```python
from build123d import *

# Parameters (mm, degrees)
SKETCH1_R           = 3.9
BOSS_EXTRUDE1_DEPTH = 50
SKETCH1_3_R         = 9.9
SKETCH1_3_R_2       = 3.9
BOSS_EXTRUDE2_DEPTH = 3
FILLET1_R           = 1


with BuildPart() as part:
    # Sketch1 → Boss-Extrude1 (new body)
    with BuildSketch(Plane.XY):
        Circle(SKETCH1_R)
    extrude(amount=BOSS_EXTRUDE1_DEPTH)

    # Sketch1_3 → Boss-Extrude2 (add)
    with BuildSketch(Plane.XY):
        Circle(SKETCH1_3_R)
        Circle(SKETCH1_3_R_2, mode=Mode.SUBTRACT)
        Circle(SKETCH1_3_R_2)
    extrude(amount=-BOSS_EXTRUDE2_DEPTH)

    # Fillet1
    fillet1_edges = [part.edges().sort_by_distance(p)[0] for p in [
        (-3.9, 0, 0),
    ]]
    fillet(fillet1_edges, radius=FILLET1_R)


solid = part.part
```
Can you work these out from the model? Positions are in its coordinate system, mm. A direction names the side the tool comes from. Give positions to 0.01 mm unless a question says otherwise; leave off trailing zeros. Write each loop counter-clockwise with the first axis right and the second up, starting at its lowest first coordinate (ties: lowest second). Pieces come first, ordered by that corner, then holes. Notation, with made-up numbers: (32.5, -1.75) - (36.5, -1.75) arc R36 cw to (36.5, 36.25) - close; hole circle Ø8 at (33, 49). An arc over 180 degrees is marked (long way). Write item = value, one per line. Start each with the question number.
1. Imagine slicing it at D-D (y = -5.5). Please give me the cut outline in (x, z).
2. Imagine slicing it at A-A (y = 0). Please give me the cut outline in (x, z), and give its area (3 significant figures).
3. Imagine slicing it at C-C (z = 18). Please give me the cut outline in (x, y), and give its area (3 significant figures).
4. Please list where these lines run through material, in increasing order: line 1 (Z direction, x = -6.5, y = -6.5); line 2 (Y direction, x = 0, z = 38.5); line 3 (X direction, y = 0.25, z = 26).
5. On a 3-axis mill with a long thin cutter (end or side, diameter ignored), from which of +Z, -Z, +X, -X, +Y, -Y can I reach the whole of each face in a straight line? I mean faces 1 (the face through (-5, -2, 0)), 2 (the face through (9.443, 2.974, -1.479)). Say none if no direction works.
6. For pin 1 (2 mm diameter, centred on x = 3, z = 19, fed in from +Y); pin 2 (3 mm diameter, centred on x = -3, z = 39, fed in from +Y); pin 3 (6 mm diameter, centred on y = 6, z = 42, fed in from -X), each with a flat end and sliding along its axis, tell me the tip position at first contact or that it passes through.
Worked answers:
q1.outline = (-8.23, -3) - (8.23, -3) - (8.23, 0) - (-8.23, 0) - close
q2.outline = (-9.9, -3) - (9.9, -3) - (9.9, 0) - (4.9, 0) arc R1 cw to (3.9, 1) - (3.9, 50) - (-3.9, 50) - (-3.9, 1) arc R1 cw to (-4.9, 0) - (-9.9, 0) - close
q2.area = 450 mm2
q3.outline = circle Ø7.8 at (0, 0)
q3.area = 47.8 mm2
q4.line_1 = -3 to 0
q4.line_2 = -3.9 to 3.9
q4.line_3 = -3.89 to 3.89
q5.face_1 = +Z
q5.face_2 = +Z, -Z
q6.pin_1 = 3.35
q6.pin_2 = 3.6
q6.pin_3 = -2.49
